Can you work these out from the model? Positions are in its coordinate system, mm. Face numbers are marked on the shaded views. A direction names the side the tool comes from. Coordinates: 2 decimals unless noted, no trailing zeros. Order: outer loops, then holes, each group sorted by start corner. A loop starts at its lowest first (then second) coordinate and runs counter-clockwise, first axis right, second up. Notation, with made-up numbers: (41.5, -29) -> (60.5, -29) arc R22 ccw to (60.5, -7) -> close; hole circle Ø9 at (71.25, -9). An arc over 180 degrees is marked (long way). Return JSON: item names as keys, results as strings. Group by question number.
1) For the marked faces 1 and 2, which set-ups out of +Z, -Z, +X, -X, +Y, -Y let a thin tool reach every point of the face, with its end or its side?
2) If we section it at B-B, the plane y = 0: Please give me the cut outline in (x, z), then the cut area to 3 significant figures.
3) If I drill on probe 1 along Z at (x, y) = (-23, 27); probe 2 along Z at (x, y) = (0, -15); probe 3 along X at (y, z) = (-3, -28), over which ranges is the centre line in solid material (lowest first)? Write a range as from..to.
4) If we section it at C-C, the plane z = 2.5: Please give me the cut outline in (x, y), then the cut area to 3 significant figures.
5) If we section it at A-A, the plane x = 0: Please give me the cut outline in (y, z), then the cut area to 3 significant figures.
6) If we section it at D-D, the plane y = -17.5: Please give me the cut outline in (x, z), then the cut area to 3 significant figures.
7) For pin 1 (10 mm diameter, centred on x = -28, z = -6, fed in from -Y); pin 2 (2 mm diameter, centred on x = 16, y = -25.5, fed in from -Z); pin 3 (12 mm diameter, centred on y = -21.5, z = 1, fed in from +X), each with a flat end and sliding along its axis, tell me the tip position at first contact or that it passes through.
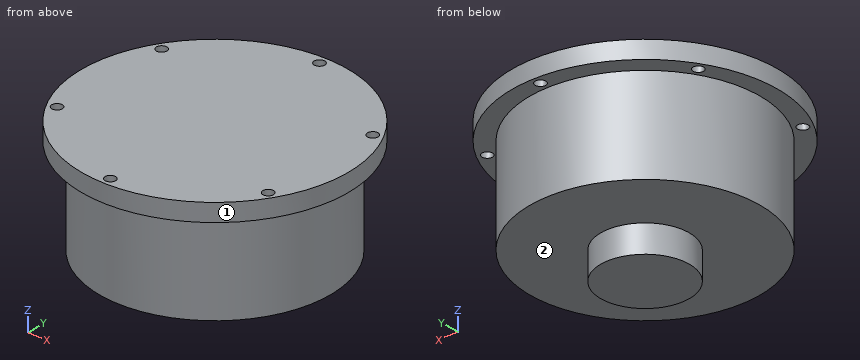
from build123d import *

# Parameters (mm, degrees)
SKETCH1_R           = 37.5
SKETCH1_R_2         = 1.5
BOSS_EXTRUDE1_DEPTH = 5
SKETCH2_R           = 32.5
BOSS_EXTRUDE2_DEPTH = 27
SKETCH3_R           = 12.5
BOSS_EXTRUDE3_DEPTH = 7.75


with BuildPart() as part:
    # Sketch1 → Boss-Extrude1 (new body)
    with BuildSketch(Plane.XY):
        Circle(SKETCH1_R)
        with Locations((0, 35)):
            Circle(SKETCH1_R_2, mode=Mode.SUBTRACT)
        with Locations((30.310889132, 17.5)):
            Circle(SKETCH1_R_2, mode=Mode.SUBTRACT)
        with Locations((30.310889132, -17.5)):
            Circle(SKETCH1_R_2, mode=Mode.SUBTRACT)
        with Locations((0, -35)):
            Circle(SKETCH1_R_2, mode=Mode.SUBTRACT)
        with Locations((-30.310889132, -17.5)):
            Circle(SKETCH1_R_2, mode=Mode.SUBTRACT)
        with Locations((-30.310889132, 17.5)):
            Circle(SKETCH1_R_2, mode=Mode.SUBTRACT)
    extrude(amount=BOSS_EXTRUDE1_DEPTH)

    # Sketch2 → Boss-Extrude2 (add)
    with BuildSketch(Plane(origin=(0, 0, 0), x_dir=(-1, 0, 0), z_dir=(0, 0, -1))):
        Circle(SKETCH2_R)
    extrude(amount=BOSS_EXTRUDE2_DEPTH)

    # Sketch3 → Boss-Extrude3 (add)
    with BuildSketch(Plane(origin=(0, 0, -27), x_dir=(-1, 0, 0), z_dir=(0, 0, -1))):
        Circle(SKETCH3_R)
    extrude(amount=BOSS_EXTRUDE3_DEPTH)


solid = part.part
Result sheet:
{
 "1": {"face 1": "+Z, -Z", "face 2": "-Z"},
 "2": {"outline": "(-37.5, 0) -> (-32.5, 0) -> (-32.5, -27) -> (-12.5, -27) -> (-12.5, -34.75) -> (12.5, -34.75) -> (12.5, -27) -> (32.5, -27) -> (32.5, 0) -> (37.5, 0) -> (37.5, 5) -> (-37.5, 5) -> close", "area": "2,320 mm2"},
 "3": {"probe 1": "z = 0..5", "probe 2": "z = -27..5", "probe 3": "x = -12.13..12.13"},
 "4": {"outline": "circle Ø75 at (0, 0); hole circle Ø3 at (-30.31, -17.5); hole circle Ø3 at (-30.31, 17.5); hole circle Ø3 at (0, -35); hole circle Ø3 at (0, 35); hole circle Ø3 at (30.31, -17.5); hole circle Ø3 at (30.31, 17.5)", "area": "4,380 mm2"},
 "5": {"outline": "(-37.5, 0) -> (-36.5, 0) -> (-36.5, 5) -> (-37.5, 5) -> close; (-33.5, 0) -> (-32.5, 0) -> (-32.5, -27) -> (-12.5, -27) -> (-12.5, -34.75) -> (12.5, -34.75) -> (12.5, -27) -> (32.5, -27) -> (32.5, 0) -> (33.5, 0) -> (33.5, 5) -> (-33.5, 5) -> close; (36.5, 0) -> (37.5, 0) -> (37.5, 5) -> (36.5, 5) -> close", "area": "2,290 mm2"},
 "6": {"outline": "(-33.17, 0) -> (-31.81, 0) -> (-31.81, 5) -> (-33.17, 5) -> close; (-28.81, 0) -> (-27.39, 0) -> (-27.39, -27) -> (27.39, -27) -> (27.39, 0) -> (28.81, 0) -> (28.81, 5) -> (-28.81, 5) -> close; (31.81, 0) -> (33.17, 0) -> (33.17, 5) -> (31.81, 5) -> close", "area": "1,780 mm2"},
 "7": {"pin 1": "stops at y = -22.96", "pin 2": "stops at z = -27", "pin 3": "stops at x = 34.15"}
}
